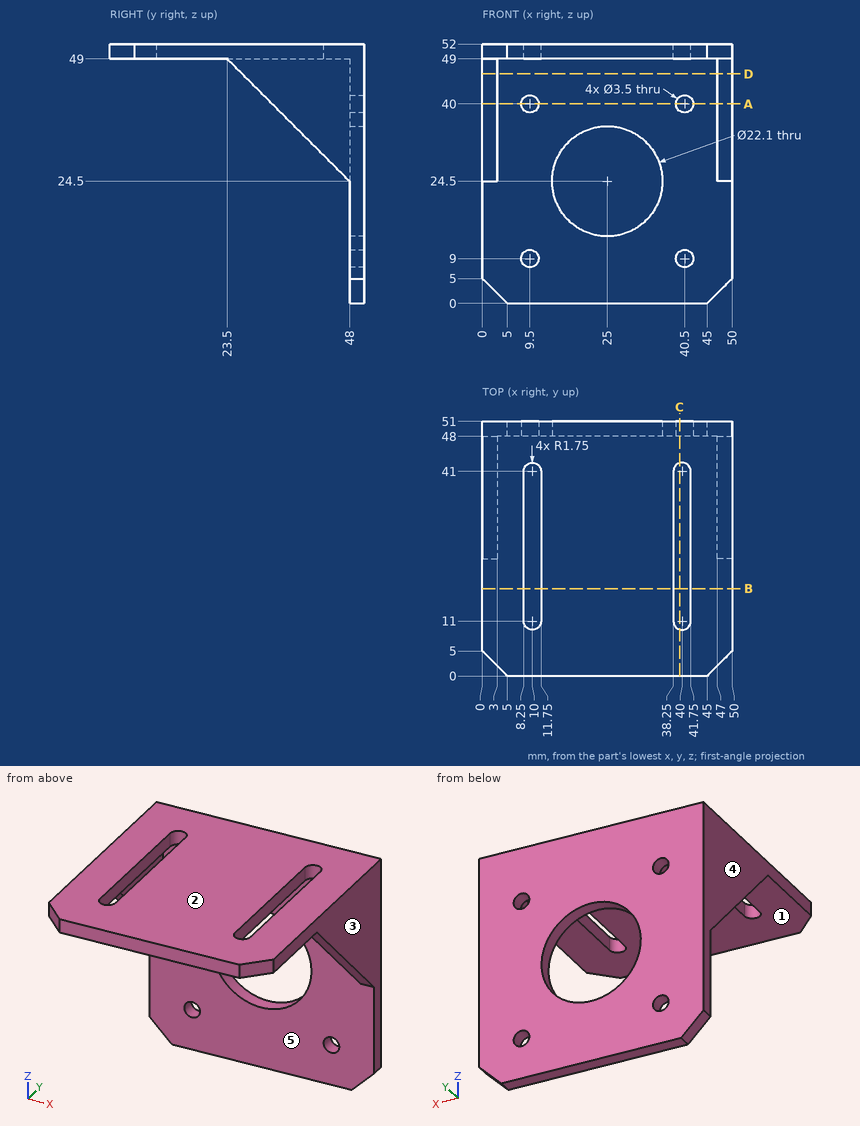
Here's the drawing with two shaded views (mm, measured from the low corner). I have some questions. A direction names the side the tool comes from. Coordinates: 2 decimals unless noted, no trailing zeros. Loops run counter-clockwise (first coordinate to the right, second up) from the corner with the lowest first, then second, coordinate; pieces in that order, holes last. Notation, with made-up numbers: (58, 21) -> (114, 21) arc R9 ccw to (114, 31) -> close; hole circle Ø3 at (25, 73.25). An arc over 180 degrees is marked (long way). Answer as a JSON object with one key per item and string values.
1) Imagine slicing it at C-C (x = 39.5). Please give me the cut outline in (y, z).
Results:
{"outline": "(0, 49) -> (9.32, 49) -> (9.32, 52) -> (0, 52) -> close; (42.68, 49) -> (48, 49) -> (48, 41.44) -> (51, 41.44) -> (51, 52) -> (42.68, 52) -> close; (48, 0) -> (51, 0) -> (51, 7.56) -> (48, 7.56) -> close; (48, 10.44) -> (51, 10.44) -> (51, 38.56) -> (48, 38.56) -> close"}
2) Imagine slicing it at B-B (y = 17.5). Please give me the cut outline in (x, z), then the cut area to 3 significant figures.
Results:
{"outline": "(0, 49) -> (8.25, 49) -> (8.25, 52) -> (0, 52) -> close; (11.75, 49) -> (38.25, 49) -> (38.25, 52) -> (11.75, 52) -> close; (41.75, 49) -> (50, 49) -> (50, 52) -> (41.75, 52) -> close", "area": "129 mm^2"}
3) If I drill on line 1 (X direction, y = 49, z = 9); line 2 (X direction, y = 49, z = 24.5); line 3 (Z direction, x = 19, y = 27.5), over which ranges is the centre line in solid material (lowest first)?
Results:
{"line 1": "x = 0 to 7.75, 11.25 to 38.75, 42.25 to 50", "line 2": "x = 0 to 13.95, 36.05 to 50", "line 3": "z = 49 to 52"}
4) Thinking about a two-plate mould opening in X: for the marked faces 3, 4 and 5, which applies, pulls with the +X half, pulls with the -X half, needs draft (parallel to the pull), parting line crosses it, or undercut?
Results:
{"face 3": "pulls with the +X half", "face 4": "pulls with the -X half", "face 5": "undercut"}
5) Imagine slicing it at D-D (z = 46). Please give me the cut outline in (x, y).
Results:
{"outline": "(0, 26.5) -> (3, 26.5) -> (3, 48) -> (47, 48) -> (47, 26.5) -> (50, 26.5) -> (50, 51) -> (0, 51) -> close"}
6) For the marked faces 1 and 2, which set-ups out of +Z, -Z, +X, -X, +Y, -Y let a thin tool reach every point of the face, with its end or its side?
Results:
{"face 1": "-Z, -Y", "face 2": "+Z, +X, -X, +Y, -Y"}
7) For P1, Ø4.5, axis at x = 40.5, z = 9, coming from the -Y side; P2, Ø14.5, axis at x = 37.5, y = 19.5, coming from the -Z side, each with a flat end and sliding along its axis, tell me the tip position at first contact or that it passes through.
Results:
{"P1": "stops at y = 48", "P2": "stops at z = 49"}
8) Imagine slicing it at A-A (z = 40). Please give me the cut outline in (x, y).
Results:
{"outline": "(0, 32.5) -> (3, 32.5) -> (3, 48) -> (7.75, 48) -> (7.75, 51) -> (0, 51) -> close; (11.25, 48) -> (38.75, 48) -> (38.75, 51) -> (11.25, 51) -> close; (42.25, 48) -> (47, 48) -> (47, 32.5) -> (50, 32.5) -> (50, 51) -> (42.25, 51) -> close"}
